```python
from build123d import *

# Parameters (mm, degrees)
F0_R     = 1.4
F3_DEPTH = 1.5
F4_R     = 1.6
F4_R_2   = 1.4
F5_DEPTH = 1
F6_R     = 0.85
F7_DEPTH = 2


with BuildPart() as f2:
    # F1 (on Front) → F2 (revolve)
    with BuildSketch(Plane.XZ):
        with BuildLine():
            Line((-1.4, 0), (0, 0))
            Line((0, 0), (0, 2))
            Line((0, 2), (-1.3, 2))
            ThreePointArc((-1.3, 2), (-1.6800297616, 1.0165014881), (-1.4, 0))
        make_face()
    revolve(axis=Axis((0, 0, 1), (0, 0, 1)))

    # F0 (on Top) → F3 (join)
    with BuildSketch(Plane.XY):
        Circle(F0_R)
    extrude(amount=-F3_DEPTH)

    # F4 (on face) → F5 (join)
    with BuildSketch(Plane(origin=(0, 0, -1.5), x_dir=(1, 0, 0), z_dir=(0, 0, -1))):
        with BuildLine():
            ThreePointArc((-8, 0), (-8.3079577623, 1.323974543), (-9.168605727, 2.3761302609))
            ThreePointArc((-9.168605727, 2.3761302609), (-14, 0), (-9.168605727, -2.3761302609))
            ThreePointArc((-9.168605727, -2.3761302609), (-8.3079577623, -1.323974543), (-8, 0))
        make_face()
        with Locations((-11, 0)):
            Circle(F4_R, mode=Mode.SUBTRACT)
        with BuildLine():
            ThreePointArc((-1.7369017855, -2.3223204317), (1.2986502266, -2.592972732), (2.9, 0))
            ThreePointArc((2.9, 0), (1.2986502266, 2.592972732), (-1.7369017855, 2.3223204317))
            ThreePointArc((-1.7369017855, 2.3223204317), (-2.9, 0), (-1.7369017855, -2.3223204317))
        make_face()
        Circle(F4_R_2, mode=Mode.SUBTRACT)
        with BuildLine():
            ThreePointArc((-1.7369017855, -2.3223204317), (-2.9, 0), (-1.7369017855, 2.3223204317))
            ThreePointArc((-1.7369017855, 2.3223204317), (-5.4618104216, 1.0984045098), (-9.168605727, 2.3761302609))
            ThreePointArc((-9.168605727, 2.3761302609), (-8.3079577623, 1.323974543), (-8, 0))
            ThreePointArc((-8, 0), (-8.3079577623, -1.323974543), (-9.168605727, -2.3761302609))
            ThreePointArc((-9.168605727, -2.3761302609), (-5.4618104216, -1.0984045098), (-1.7369017855, -2.3223204317))
        make_face()
        Circle(F4_R_2)
    extrude(amount=F5_DEPTH)

    # F6 (on face) → F7 (cut)
    with BuildSketch(Plane.XY.offset(2)):
        Circle(F6_R)
    extrude(amount=-F7_DEPTH, mode=Mode.SUBTRACT)


solid = f2.part
```
Could you check a few things on this model? Use its own coordinates, in mm. A direction names the side the tool comes from. Give positions to 0.01 mm unless a question says otherwise; leave off trailing zeros. Loops run counter-clockwise (first coordinate to the right, second up) from the corner with the lowest first, then second, coordinate; pieces in that order, holes last. Notation, with made-up numbers: (-12.75, -34.5) -> (-0.75, -34.5) arc R11 cw to (-0.75, -28.5) -> close; hole circle Ø1 at (31.5, 23). An arc over 180 degrees is marked (long way). Put each result on its own line as item: value.
(1) Imagine slicing it at A-A on x = -11. Write out the boundary of the cut face in (y, z), plus the area to 3 significant figures.
Computed:
outline: (-3, -2.5) -> (-1.6, -2.5) -> (-1.6, -1.5) -> (-3, -1.5) -> close; (1.6, -2.5) -> (3, -2.5) -> (3, -1.5) -> (1.6, -1.5) -> close
area: 2.80 mm^2
(2) I'm going to push flat-ended pins straight in: pin 1 Ø1.8 at (x, y) = (-4.5, 0.5) entering from +Z; pin 2 Ø1 at (x, y) = (0, 0) entering from +Z; pin 3 Ø1.5 at (y, z) = (1, 0) entering from +X; pin 4 Ø0.8 at (x, y) = (0, 0.5) entering from +Z. Where does each tip first touch, or does it pass through?
Computed:
pin 1: z = -1.5
pin 2: z = 0
pin 3: x = 1.56
pin 4: z = 2
(3) Imagine slicing it at B-B on y = 0.35. Write out the boundary of the cut face in (x, z).
Computed:
outline: (-13.98, -2.5) -> (-12.56, -2.5) -> (-12.56, -1.5) -> (-13.98, -1.5) -> close; (-9.44, -2.5) -> (2.88, -2.5) -> (2.88, -1.5) -> (1.36, -1.5) -> (1.36, 0) arc R1.65 ccw to (1.25, 2) -> (0.77, 2) -> (0.77, 0) -> (-0.77, 0) -> (-0.77, 2) -> (-1.25, 2) arc R1.65 ccw to (-1.36, 0) -> (-1.36, -1.5) -> (-9.44, -1.5) -> close
(4) Please list where these lines run through material, in increasing order: probe 1 along Y at (x, z) = (-11, -1.8); probe 2 along X at (y, z) = (0.1, -0.65); probe 3 along Y at (x, z) = (0, 0.5). Write a range as [from, to].
Computed:
probe 1: [-3, -1.6], [1.6, 3]
probe 2: [-1.4, 1.4]
probe 3: [-1.63, -0.85], [0.85, 1.63]
(5) Thinking about a two-plate mould opening in Y: for faces 3 (the face through (-12.6, -0.07, -1.99)), 4 (the face through (-1.4, 0.06, -0.74)), 5 (the face through (-0.18, -0.83, 1.01)), 6 (the face through (-6, 0, -2.5)), which applies, pulls with the +Y half, pulls with the -Y half, needs draft (parallel to the pull), parting line crosses it, or undercut?
Computed:
face 3: undercut
face 4: parting line crosses it
face 5: undercut
face 6: needs draft
(6) For faces 1 (the face through (-5.4, -1.1, -2)), 2 (the face through (0, 0, 0)), which set-ups out of +Z, -Z, +X, -X, +Y, -Y let a thin tool reach every point of the face, with its end or its side?
Computed:
face 1: +Z, -Z, -Y
face 2: +Z
(7) Imagine slicing it at D-D on z = 0.55. Write out the boundary of the cut face in (x, y), plus the area to 3 significant figures.
Computed:
outline: circle Ø3.28 at (0, 0); hole circle Ø1.7 at (0, 0)
area: 6.16 mm^2
(8) Imagine slicing it at C-C on x = 0. Write out the boundary of the cut face in (y, z).
Computed:
outline: (-2.9, -2.5) -> (2.9, -2.5) -> (2.9, -1.5) -> (1.4, -1.5) -> (1.4, 0) arc R1.68 ccw to (1.3, 2) -> (0.85, 2) -> (0.85, 0) -> (-0.85, 0) -> (-0.85, 2) -> (-1.3, 2) arc R1.68 ccw to (-1.4, 0) -> (-1.4, -1.5) -> (-2.9, -1.5) -> close
